from build123d import *

# Parameters (mm, degrees)
SKETCH1_W           = 40
SKETCH1_H           = 30
BOSS_EXTRUDE1_DEPTH = 3
BOSS_EXTRUDE2_DEPTH = 2
FILLET1_R           = 2


with BuildPart() as part:
    # Sketch1 → Boss-Extrude1 (new body)
    with BuildSketch(Plane(origin=(0, 0, 0), x_dir=(0, 0, -1), z_dir=(1, 0, 0))):
        Rectangle(SKETCH1_W, SKETCH1_H)
    extrude(amount=BOSS_EXTRUDE1_DEPTH)

    # Sketch2 → Boss-Extrude2 (add)
    with BuildSketch(Plane(origin=(3, 0, 0), x_dir=(0, 0, -1), z_dir=(1, 0, 0))):
        Polygon((18, 0), (18, 13), (-13.768503326, 13), (-18, 13), (-18, 10), (-15, 10), (15, 10), (15, 0), align=None)
    extrude(amount=BOSS_EXTRUDE2_DEPTH)

    # Fillet1
    # the kernel refuses this fillet: 2 mm, written as the material it takes off along each edge
    with BuildSketch(Plane(origin=(5, 10, -15), x_dir=(-1, 0, 0), z_dir=(0, 0, 1))) as fillet1_piece_1:
        with BuildLine():
            CenterArc((FILLET1_R, -FILLET1_R), FILLET1_R, 90, 90)
            Line((0, -FILLET1_R), (0, 0))
            Line((0, 0), (FILLET1_R, 0))
        make_face()
    extrude(amount=38, mode=Mode.SUBTRACT)
    with BuildSketch(Plane(origin=(5, 13, 23), x_dir=(-1, 0, 0), z_dir=(0, 0, -1))) as fillet1_piece_2:
        with BuildLine():
            CenterArc((FILLET1_R, -FILLET1_R), FILLET1_R, 90, 90)
            Line((0, -FILLET1_R), (0, 0))
            Line((0, 0), (FILLET1_R, 0))
        make_face()
    extrude(amount=46, mode=Mode.SUBTRACT)
    with BuildSketch(Plane(origin=(5, 10, -15), x_dir=(-1, 0, 0), z_dir=(0, -1, 0))) as fillet1_piece_3:
        with BuildLine():
            CenterArc((FILLET1_R, FILLET1_R), FILLET1_R, 180, 90)
            Line((0, FILLET1_R), (0, 0))
            Line((0, 0), (FILLET1_R, 0))
        make_face()
    extrude(amount=15, mode=Mode.SUBTRACT)
    with BuildSketch(Plane(origin=(5, -5, -18), x_dir=(-1, 0, 0), z_dir=(0, 1, 0))) as fillet1_piece_4:
        with BuildLine():
            CenterArc((FILLET1_R, FILLET1_R), FILLET1_R, 180, 90)
            Line((0, FILLET1_R), (0, 0))
            Line((0, 0), (FILLET1_R, 0))
        make_face()
    extrude(amount=23, mode=Mode.SUBTRACT)
    with BuildSketch(Plane(origin=(5, 15, -15), x_dir=(-1, 0, 0), z_dir=(0, -1, 0))) as fillet1_piece_5a_section:
        with BuildLine():
            CenterArc((FILLET1_R, FILLET1_R), FILLET1_R, 180, 90)
            Line((0, FILLET1_R), (0, 0))
            Line((0, 0), (FILLET1_R, 0))
        make_face()
    fillet1_piece_5a = extrude(amount=20, mode=Mode.PRIVATE)
    fillet1_piece_5a = split(fillet1_piece_5a, bisect_by=Plane(origin=(4.547209771, 10, -15.452790229), z_dir=(0, 1, 0)), keep=Keep.TOP, mode=Mode.PRIVATE)
    with BuildSketch(Plane(origin=(5, 10, -20), x_dir=(-1, 0, 0), z_dir=(0, 0, 1))) as fillet1_piece_5b_section:
        with BuildLine():
            CenterArc((FILLET1_R, -FILLET1_R), FILLET1_R, 90, 90)
            Line((0, -FILLET1_R), (0, 0))
            Line((0, 0), (FILLET1_R, 0))
        make_face()
    fillet1_piece_5b = extrude(amount=43, mode=Mode.PRIVATE)
    fillet1_piece_5b = split(fillet1_piece_5b, bisect_by=Plane(origin=(4.547209771, 10.452790229, -15), z_dir=(0, 0, -1)), keep=Keep.TOP, mode=Mode.PRIVATE)
    fillet1_piece_5 = fillet1_piece_5a & fillet1_piece_5b
    add(fillet1_piece_5, mode=Mode.SUBTRACT)


solid = part.part
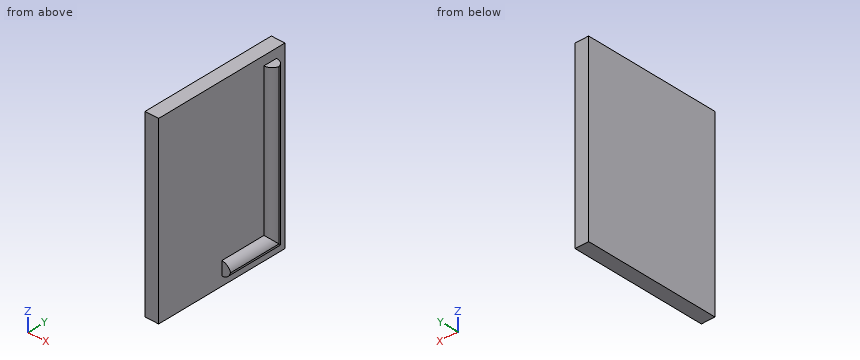
Check sheet for the modelled part. Datum: model origin and axes. Units: mm. Give positions to 0.01 mm unless a question says otherwise; leave off trailing zeros. Loops run counter-clockwise (first coordinate to the right, second up) from the corner with the lowest first, then second, coordinate; pieces in that order, holes last. Notation, with made-up numbers: M 84.5,0 L 120.5,0 A21 cw 120.5,5 Z; hole C -18,28 d2. An arc over 180 degrees is marked long. Answer as a JSON object with one key per item and string values. Group by question number.
Q1. Cross-section at C-C on x = 4. Record the cut outline in (y, z), then the cut area to 3 significant figures.
Q2. Cross-section at D-D on y = -9.75. Record the cut outline in (x, z).
Q3. Go/stop test with flat-tipped pins: P1, Ø4, axis at y = -2.5, z = 9.5, coming from the +X side; P2, Ø2, axis at x = 4.5, z = -16.5, coming from the -Y side; P3, Ø2, axis at x = 4.5, y = 12, coming from the +Z side. Record where each tip stops, or that it passes through.
Q4. Material ranges on line 1 along X through (y, z) = (9.75, 15); line 2 along Z through (x, y) = (3.15, 4.5); line 3 along Z through (x, y) = (4.65, 1.5), recorded low to high. Write a range as [from, to].
Q5. Cross-section at B-B on y = 2.5. Record the cut outline in (x, z), then the cut area to 3 significant figures.
Q6. Cross-section at A-A on z = 13.5. Record the cut outline in (x, y).
Evaluation:
{
 "1": {"outline": "M 0,-17.73 L 12.73,-17.73 L 12.73,18 L 10.27,18 L 10.27,-15.27 L 0,-15.27 Z", "area": "113 mm2"},
 "2": {"outline": "M 0,-20 L 3,-20 L 3,20 L 0,20 Z"},
 "3": {"P1": "stops at x = 3", "P2": "stops at y = 0", "P3": "stops at z = 18"},
 "4": {"line 1": "x = [0, 3]", "line 2": "z = [-17.99, -15.01]", "line 3": "z = [-17.13, -15.87]"},
 "5": {"outline": "M 0,-20 L 3,-20 L 3,-18 A2 ccw 4.94,-16.5 A2 ccw 3,-15 L 3,20 L 0,20 Z", "area": "124 mm2"},
 "6": {"outline": "M 0,-15 L 3,-15 L 3,10 A2 ccw 4.94,11.5 A2 ccw 3,13 L 3,15 L 0,15 Z"}
}
